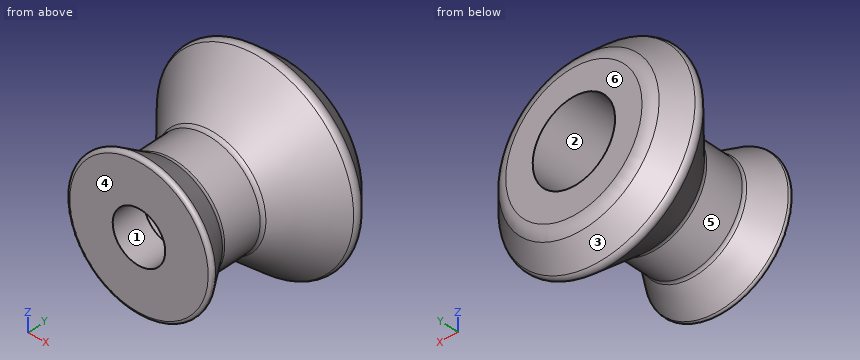
from build123d import *

# Parameters (mm, degrees)
SKETCH2_R          = 3.1496
SKETCH2_R_2        = 2.0066
CUT_EXTRUDE1_DEPTH = 9.652
SKETCH2_2_R        = 2.0066
CUT_EXTRUDE2_DEPTH = 17.363717474


with BuildPart() as part:
    # Sketch1 → Revolve1 (revolve)
    with BuildSketch(Plane.XY, mode=Mode.PRIVATE) as revolve1_sk:
        with BuildLine():
            Line((0, 0), (5.293826023, 0))
            ThreePointArc((5.293826023, 0), (5.517493338, 0.13363002), (5.505816812, 0.393913921))
            Line((5.505816812, 0.393913921), (4.173418421, 2.412699361))
            ThreePointArc((4.173418421, 2.412699361), (4.110857791, 2.54644271), (4.0894, 2.692527203))
            Line((4.0894, 2.692527203), (4.0894, 5.648040158))
            ThreePointArc((4.0894, 5.648040158), (4.122815879, 5.82924146), (4.218667369, 5.986604176))
            Line((4.218667369, 5.986604176), (7.527837593, 9.688387816))
            ThreePointArc((7.527837593, 9.688387816), (7.657085265, 10.031425293), (7.521816282, 10.37213334))
            Line((7.521816282, 10.37213334), (6.142780319, 11.861153766))
            ThreePointArc((6.142780319, 11.861153766), (5.719405756, 12.161997938), (5.21100202, 12.2682))
            Line((5.21100202, 12.2682), (0, 12.2682))
            Line((0, 12.2682), (0, 0))
        make_face()
    revolve(revolve1_sk.sketch.rotate(Axis((0, 0, 0), (0, 1, 0)), 90), axis=Axis((0, 0, 0), (0, 1, 0)))

    # Sketch2 → Cut-Extrude1 (cut)
    with BuildSketch(Plane(origin=(0, 12.2682, 0), x_dir=(1, 0, 0), z_dir=(0, 1, 0))):
        with Locations(Location((0, 0, 0), (0, 0, 270))):
            Circle(SKETCH2_R)
        with Locations(Location((0, 0, 0), (0, 0, 270))):
            Circle(SKETCH2_R_2, mode=Mode.SUBTRACT)
    extrude(amount=-CUT_EXTRUDE1_DEPTH, mode=Mode.SUBTRACT)

    # Sketch2_2 → Cut-Extrude2 (cut, through all)
    with BuildSketch(Plane(origin=(0, 12.2682, 0), x_dir=(1, 0, 0), z_dir=(0, 1, 0))):
        with Locations(Location((0, 0, 0), (0, 0, 270))):
            Circle(SKETCH2_2_R)
    extrude(amount=-CUT_EXTRUDE2_DEPTH, mode=Mode.SUBTRACT)


solid = part.part
Geometry check sheet. Reference: the model listing, model coordinates, mm. Face numbers are marked on the shaded views. A direction names the side the tool comes from. Give positions to 0.01 mm unless a question says otherwise; leave off trailing zeros. Write each loop counter-clockwise with the first axis right and the second up, starting at its lowest first coordinate (ties: lowest second). Pieces come first, ordered by that corner, then holes. Notation, with made-up numbers: (8.5, 70.5) - (41.5, 70.5) arc R15 ccw to (41.5, 80.5) - close; hole circle Ø2 at (86, 76.5). An arc over 180 degrees is marked (long way). Put each result on its own line as item: value.
1. Set-up check for the marked faces 5 and 6: record each of +Z, -Z, +X, -X, +Y, -Y from which the full face is reachable in a straight line by a thin tool's end or side.
Ans:
face 5: none
face 6: +Z, -Z, +X, -X, +Y
2. Thickness scan on line 1 (X direction, y = 4.5, z = 0); line 2 (X direction, y = 9.25, z = -1.5); line 3 (Y direction, x = 0.75, z = -2.5). Record the ranges inside material, lowest first.
Ans:
line 1: x = -4.09 to -3.15, 3.15 to 4.09
line 2: x = -6.98 to -2.77, 2.77 to 6.98
line 3: y = 0 to 2.62
3. Go/stop test with flat-tipped pins: pin 1 (5 mm diameter, centred on x = -5.5, y = 8, fed in from -Z); pin 2 (3 mm diameter, centred on x = -4, y = 2, fed in from +Z); pin 3 (3 mm diameter, centred on y = 4.5, z = 3.5, fed in from +X). Record where each tip stops, or that it passes through.
Ans:
pin 1: stops at z = -6.61
pin 2: stops at z = 4.23
pin 3: stops at x = 3.57
4. Sectioned sample at B-B, the plane z = 0. Enter the section's corners in (x, y), plus the area to 3 significant figures.
Ans:
outline: (-7.53, 9.69) - (-4.22, 5.99) arc R0.51 cw to (-4.09, 5.65) - (-4.09, 2.69) arc R0.51 cw to (-4.17, 2.41) - (-5.51, 0.39) arc R0.25 ccw to (-5.29, 0) - (-2.01, 0) - (-2.01, 2.62) - (-3.15, 2.62) - (-3.15, 12.27) - (-5.21, 12.27) arc R1.27 ccw to (-6.14, 11.86) - (-7.52, 10.37) arc R0.51 ccw to start; (2.01, 0) - (5.29, 0) arc R0.25 ccw to (5.51, 0.39) - (4.17, 2.41) arc R0.51 cw to (4.09, 2.69) - (4.09, 5.65) arc R0.51 cw to (4.22, 5.99) - (7.53, 9.69) arc R0.51 ccw to (7.52, 10.37) - (6.14, 11.86) arc R1.27 ccw to (5.21, 12.27) - (3.15, 12.27) - (3.15, 2.62) - (2.01, 2.62) - close
area: 60.9 mm²
5. Sectioned sample at D-D, the plane y = 8.25. Enter the section's corners in (x, z), plus the area to 3 significant figures.
Ans:
outline: circle Ø12.48 at (0, 0); hole circle Ø6.3 at (0, 0)
area: 91.2 mm²
6. Draft check along Z on the marked faces 1, 2, 3 and 4. Enter one of: +Z half, -Z half, draft (parallel to the pull), parting line (faces both ways), or undercut.
Ans:
face 1: undercut
face 2: undercut
face 3: parting line
face 4: draft
7. Sectioned sample at C-C, the plane y = 3.5. Enter the section's corners in (x, z).
Ans:
outline: circle Ø8.18 at (0, 0); hole circle Ø6.3 at (0, 0)
8. Sectioned sample at A-A, the plane x = 0. Enter the section's corners in (y, z), plus the area to 3 significant figures.
Ans:
outline: (0, -5.29) arc R0.25 ccw to (0.39, -5.51) - (2.41, -4.17) arc R0.51 cw to (2.69, -4.09) - (5.65, -4.09) arc R0.51 cw to (5.99, -4.22) - (9.69, -7.53) arc R0.51 ccw to (10.37, -7.52) - (11.86, -6.14) arc R1.27 ccw to (12.27, -5.21) - (12.27, -3.15) - (2.62, -3.15) - (2.62, -2.01) - (0, -2.01) - close; (0, 2.01) - (2.62, 2.01) - (2.62, 3.15) - (12.27, 3.15) - (12.27, 5.21) arc R1.27 ccw to (11.86, 6.14) - (10.37, 7.52) arc R0.51 ccw to (9.69, 7.53) - (5.99, 4.22) arc R0.51 cw to (5.65, 4.09) - (2.69, 4.09) arc R0.51 cw to (2.41, 4.17) - (0.39, 5.51) arc R0.25 ccw to (0, 5.29) - close
area: 60.9 mm²
